from build123d import *

# Parameters (mm, degrees)
F1_DEPTH = 5.08
F2_R     = 12.7
F3_DEPTH = 5.08


with BuildPart() as f1:
    # F0 (on Top) → F1 (new body)
    with BuildSketch(Plane.XY):
        with BuildLine():
            ThreePointArc((25.4, 0), (12.7, 4.8509683429), (0, 0))
            Line((0, 0), (25.4, 0))
        make_face()
        with BuildLine():
            Line((0, 127), (0, 0))
            ThreePointArc((0, 0), (12.7, 4.8509683429), (25.4, 0))
            Line((25.4, 0), (25.4, 127))
            ThreePointArc((25.4, 127), (12.7, 122.1490316571), (0, 127))
        make_face()
        with BuildLine():
            Line((25.4, 0), (0, 0))
            ThreePointArc((0, 0), (4.9228700667, -31.5892228579), (31.75, -14.1990316571))
            ThreePointArc((31.75, -14.1990316571), (30.0901912008, -6.4219017238), (25.4, 0))
        make_face()
        with BuildLine():
            ThreePointArc((31.75, 141.1990316571), (4.9228700667, 158.5892228579), (0, 127))
            Line((0, 127), (25.4, 127))
            ThreePointArc((25.4, 127), (30.0901912008, 133.4219017238), (31.75, 141.1990316571))
        make_face()
        with BuildLine():
            Line((25.4, 127), (0, 127))
            ThreePointArc((0, 127), (12.7, 122.1490316571), (25.4, 127))
        make_face()
    extrude(amount=F1_DEPTH)

    # F2 (on face) → F3 (join)
    with BuildSketch(Plane.XY.offset(5.08)):
        with Locations((12.7, -14.1990316571)):
            Circle(F2_R)
        with Locations((12.7, 141.1990316571)):
            Circle(F2_R)
    extrude(amount=F3_DEPTH)


solid = f1.part
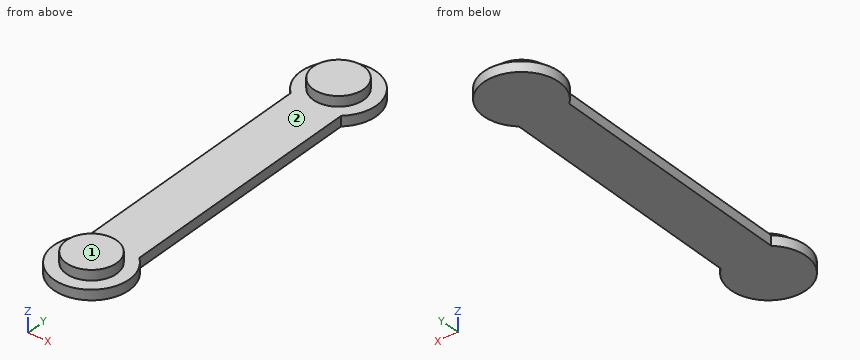
Work out the finished part from the listing and answer in its coordinate system (mm). Face numbers are marked on the shaded views. Coordinates: 2 decimals unless noted, no trailing zeros. Write each loop counter-clockwise with the first axis right and the second up, starting at its lowest first coordinate (ties: lowest second). Pieces come first, ordered by that corner, then holes. Notation, with made-up numbers: M 47.5,13.5 L 65.5,13.5 A25 ccw 65.5,34.5 Z; hole C -3,78.5 d6. An arc over 180 degrees is marked long. Use one line per item in the form item = value. Start each with the question number.
1. Each of these flat-tipped pins is pushed along its axis until it touches: P1, Ø5, axis at y = 126, z = 2.5, coming from the +X side; P2, Ø1, axis at y = 133, z = 8, coming from the +X side; P3, Ø3, axis at x = 9, z = 4, coming from the -Y side. Where does it stop, or does it pass through?
2. The part is cut by section B-B (z = 1.75). Give the vertices of the cut face in (x, y).
3. The mould has two halves that part along Y. Classify the marked faces 1 and 2: released by +Y, released by -Y, zero draft, split by the parting line, or undercut.
4. The part is cut by section A-A (x = 6.5). Give the vertices of the cut face in (y, z), plus the area to 3 significant figures.
5. The part is cut by section C-C (y = 25). Give the vertices of the cut face in (x, z), plus the area to 3 significant figures.
6. Straight lines are drawn through the part: probe 1 along Y at (x, z) = (12, 9.25); probe 2 along Z at (x, y) = (13.5, 55); probe 3 along X at (y, z) = (50, 3.5). For each, find the intervals that lie inside material, in ascending order. Write a range as from..to.
Evaluation:
q1.P1 = 26.9
q1.P2 = 22.8
q1.P3 = -33.12
q2.outline = M 0,0 A19.05 ccw long 25.4,0 L 25.4,127 A19.05 ccw long 0,127 Z
q3.face_1 = zero draft
q3.face_2 = undercut
q4.outline = M -32.21,0 L 159.21,0 L 159.21,5.08 L 152.28,5.08 L 152.28,10.16 L 130.12,10.16 L 130.12,5.08 L -3.12,5.08 L -3.12,10.16 L -25.28,10.16 L -25.28,5.08 L -32.21,5.08 Z
q4.area = 1,200 mm^2
q5.outline = M 0,0 L 25.4,0 L 25.4,5.08 L 0,5.08 Z
q5.area = 129 mm^2
q6.probe_1 = -26.88..-1.52, 128.52..153.88
q6.probe_2 = 0..5.08
q6.probe_3 = 0..25.4
